Could you check a few things on this drawing? It's one solid part, dimensions in mm from its lowest x, y, z. A direction names the side the tool comes from. Give positions to 0.01 mm unless a question says otherwise; leave off trailing zeros. Loops run counter-clockwise (first coordinate to the right, second up) from the corner with the lowest first, then second, coordinate; pieces in that order, holes last.
1. Imagine slicing it at D-D (y = 6.25). List the corners of the cut face in (x, z) for me.
2. For P1, Ø3, axis at y = 3, z = 12, coming from the -X side; P2, Ø5.5, axis at x = 6.5, y = 7.5, coming from the -Z side, each with a flat end and sliding along its axis, tell me the tip position at first contact or that it passes through.
3. Thinking about a two-plate mould opening in Y: for the marked faces 3, 4, 5 and 6, which applies, +Y half, -Y half, draft (parallel to the pull), parting line (faces both ways), or undercut?
4. Imagine slicing it at B-B (x = 2.5). List the corners of the cut face in (y, z) for me.
5. I need wall thicknesses on line 1 along Y through (x, z) = (3.5, 15.4); line 2 along Y through (x, z) = (4.5, 15.25); line 3 along Y through (x, z) = (11.35, 3.5). Which ranges of each line are inside material? Lowest first, please.
6. For the marked faces 1 and 2, which set-ups out of +Z, -Z, +X, -X, +Y, -Y let a thin tool reach every point of the face, with its end or its side?
7. Imagine slicing it at A-A (y = 11.5). List the corners of the cut face in (x, z) for me.
8. Imagine slicing it at C-C (z = 1.5). List the corners of the cut face in (x, y) for me, plus the area to 3 significant figures.
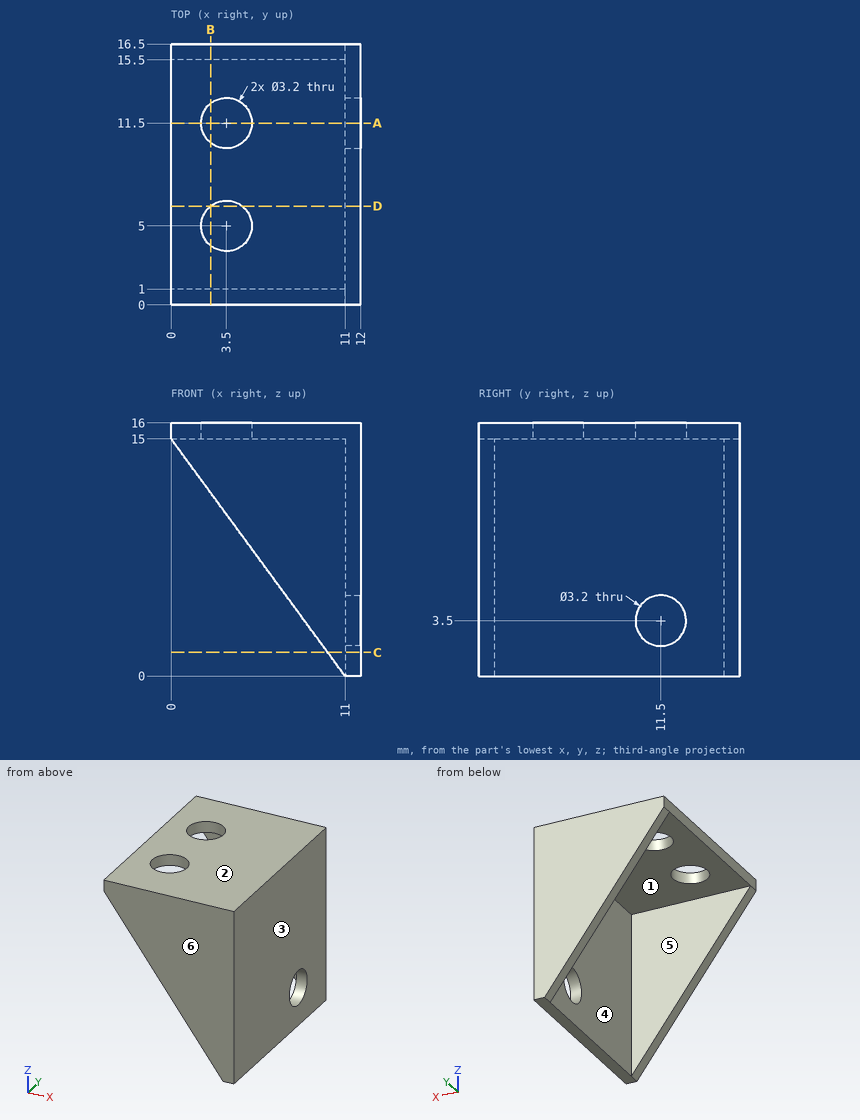
Derived:
1. outline: (0, 15) - (2.5, 15) - (2.5, 16) - (0, 16) - close; (4.5, 15) - (11, 15) - (11, 0) - (12, 0) - (12, 16) - (4.5, 16) - close
2. P1: stops at x = 11
2. P2: stops at z = 15
3. face 3: draft
3. face 4: undercut
3. face 5: undercut
3. face 6: -Y half
4. outline: (0, 11.59) - (1, 11.59) - (1, 15) - (3.75, 15) - (3.75, 16) - (0, 16) - close; (6.25, 15) - (10.25, 15) - (10.25, 16) - (6.25, 16) - close; (12.75, 15) - (15.5, 15) - (15.5, 11.59) - (16.5, 11.59) - (16.5, 16) - (12.75, 16) - close
5. line 1: y = 0 to 3.4, 6.6 to 9.9, 13.1 to 16.5
5. line 2: y = 0 to 3.75, 6.25 to 10.25, 12.75 to 16.5
5. line 3: y = 0 to 9.9, 13.1 to 16.5
6. face 1: -Z, -X
6. face 2: +Z, +X, -X, +Y, -Y
7. outline: (0, 15) - (1.9, 15) - (1.9, 16) - (0, 16) - close; (5.1, 15) - (11, 15) - (11, 5.1) - (12, 5.1) - (12, 16) - (5.1, 16) - close; (11, 0) - (12, 0) - (12, 1.9) - (11, 1.9) - close
8. outline: (9.9, 0) - (12, 0) - (12, 16.5) - (9.9, 16.5) - (9.9, 15.5) - (11, 15.5) - (11, 1) - (9.9, 1) - close
8. area: 18.7 mm2
